Source: three-view drawing plus pictorial views. Frame: mm from the lowest corner of the part. Give positions to 0.01 mm unless a question says otherwise; leave off trailing zeros. Order: outer loops, then holes, each group sorted by start corner. A loop starts at its lowest first (then second) coordinate and runs counter-clockwise, first axis right, second up. Notation, with made-up numbers: (4.5, -28) -> (37.5, -28) arc R18 ccw to (37.5, 1) -> close; hole circle Ø3 at (-2.75, 52). An arc over 180 degrees is marked (long way). Answer in a Markdown table with one row per item. Add a question column.
Q1. Cut plane C-C on y = 10.5. Count the separate pieces of the cut face and the enclosed holes in it, and give its area (3 significant figures).
Q2. Cut plane B-B on z = 155. Return the cut outline in (x, y).
Q3. Pull-direction query (Z, two-part tool) for the marked faces 1, 2 and 3; classes: +Z half, -Z half, draft (parallel to the pull), parting line (faces both ways), or undercut.
Q4. Cut plane D-D on x = 50. Return the cut outline in (y, z), and give its area (3 significant figures).
Q5. Cut plane A-A on z = 90. Return the cut outline in (x, y), and give its area (3 significant figures).
Q6. Contact query for a flat-ended pin moving along its axis: P1, Ø8, axis at x = 22, y = 5.5, coming from the -Z side. Output: stop coordinate, or through.
Q7. Line query: line 1 along Z through (x, y) = (90, 14.75); line 2 along Z through (x, y) = (26, 9); line 3 along X through (y, z) = (3.25, 141). Output: solid intervals per line, ascending. Write a range as from..to.
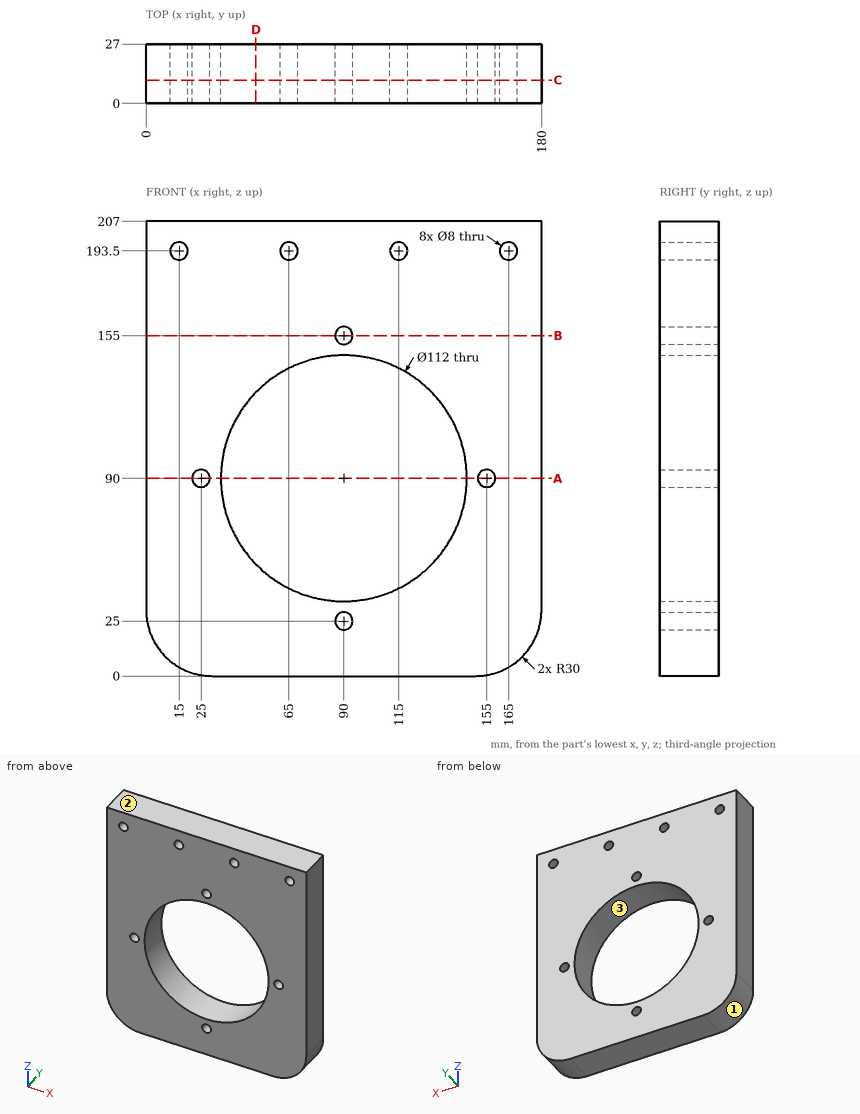
Completed:
| question | item | result |
|---|---|---|
| 1 | separate pieces | 1 |
| 1 | enclosed holes | 9 |
| 1 | area | 26,600 mm² |
| 2 | outline | (0, 0) -> (86, 0) -> (86, 27) -> (0, 27) -> close; (94, 0) -> (180, 0) -> (180, 27) -> (94, 27) -> close |
| 3 | face 1 | -Z half |
| 3 | face 2 | +Z half |
| 3 | face 3 | undercut |
| 4 | outline | (0, 0) -> (27, 0) -> (27, 50.81) -> (0, 50.81) -> close; (0, 129.19) -> (27, 129.19) -> (27, 207) -> (0, 207) -> close |
| 4 | area | 3,470 mm² |
| 5 | outline | (0, 0) -> (21, 0) -> (21, 27) -> (0, 27) -> close; (29, 0) -> (34, 0) -> (34, 27) -> (29, 27) -> close; (146, 0) -> (151, 0) -> (151, 27) -> (146, 27) -> close; (159, 0) -> (180, 0) -> (180, 27) -> (159, 27) -> close |
| 5 | area | 1,400 mm² |
| 6 | P1 | stops at z = 0.27 |
| 7 | line 1 | z = 0..21, 29..34, 146..151, 159..207 |
| 7 | line 2 | z = 0.27..86.13, 93.87..207 |
| 7 | line 3 | x = 0..66.87, 113.13..180 |
